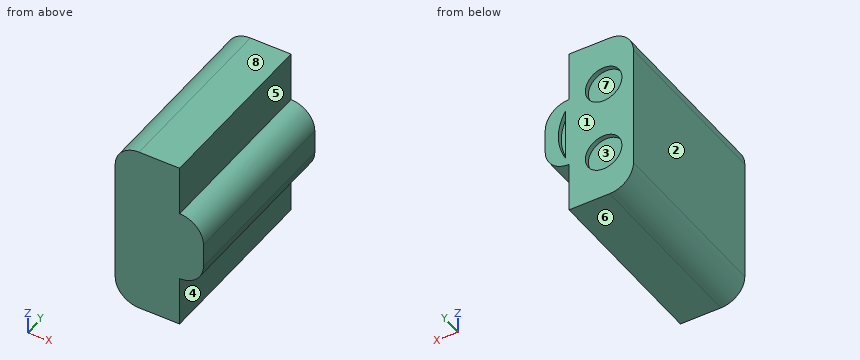
Autodesk Inventor part; units mm, degrees
ref_plane "YZ Plane" through (0, 0, 0) normal (1, 0, 0) x (0, 1, 0)
ref_plane "XZ Plane" through (0, 0, 0) normal (0, 1, 0) x (-1, 0, 0)
ref_plane "XY Plane" through (0, 0, 0) normal (0, 0, 1) x (1, 0, 0)
sketch "Esquisse1" plane through (0, 0, 0) normal (0, 1, 0) x (-1, 0, 0)
  line L0 (0, 0) -> (27, 0)
  line L1 (27, 0) -> (27, -72)
  line L2 (27, -72) -> (0, -72)
  line L3 (0, -72) -> (0, 0)
  line L4 (0, -21) -> (-10, -21)
  line L5 (-10, -21) -> (-10, -51)
  line L6 (-10, -51) -> (0, -51)
  line L7 (0, -51) -> (0, -21)
  point P0 (0, -36)
  dimension "d0" = 27
  dimension "d1" = 72
  dimension "d2" = 30
  dimension "d3" = 10
extrude "Extrusion1" add sketch "Esquisse1" along normal blind 75
sketch "Esquisse2" plane through (0, 75, 0) normal (0, 1, 0) x (1, 0, 0)
  line L0 (0, 21) -> (10, 21) construction
  line L1 (10, 21) -> (10, 51) construction
  line L2 (10, 51) -> (0, 51) construction
  line L3 (0, 51) -> (0, 72) construction
  line L4 (0, 72) -> (-27, 72) construction
  line L5 (-27, 72) -> (-27, 0) construction
  line L6 (-27, 0) -> (0, 0) construction
  line L7 (0, 0) -> (0, 21) construction
  line L8 (-27, 72) -> (-27, 0) construction
  line L9 (-27, 72) -> (-27, 0) construction
  line L10 (-27, 36) -> (10, 36) construction
  circle A0 centre (-14.5005, 20.2664) radius 7.6563
  circle A1 centre (-14.5005, 51.7336) radius 7.6563
  line L11 (1.4504, 25.5678) -> (1.4504, 47.6136)
  line L12 (1.4504, 25.5678) -> (7.5686, 36) construction
  line L13 (7.5686, 36) -> (1.4504, 47.6136) construction
  spline S0 degree 2 poles (1.4504, 25.5678) (7.5686, 36) (1.4504, 47.6136) knots 1 1 1 2 2 2
  dimension "d28" = 15.3126
extrude "Extrusion2" cut sketch "Esquisse2" against normal blind 2
fillet "Congé1" radius 10 2 edges at (-27, 37.5, -72) (-27, 37.5, 0)
fillet "Congé2" radius 10 2 edges at (10, 37.5, -51) (10, 37.5, -21)
ref_plane "Plan de construction1" through (0, 60, 0) normal (0, 1, 0) x (1, 0, 0)
sketch "Esquisse3" plane through (0, 0, -72) normal (0, 0, -1) x (-1, 0, 0)
  point P0 (0, 0)
sketch "Esquisse4" plane through (0, 60, 0) normal (0, 1, 0) x (1, 0, 0)
  arc A0 (0, 21) -> (10, 31) centre (0, 31) ccw
  line L0 (10, 31) -> (10, 41)
  arc A1 (10, 41) -> (0, 51) centre (0, 41) ccw
  line L1 (0, 51) -> (0, 72)
  line L2 (0, 72) -> (-17, 72)
  arc A2 (-17, 72) -> (-27, 62) centre (-17, 62) ccw
  line L3 (-27, 62) -> (-27, 10)
  arc A3 (-27, 10) -> (-17, 0) centre (-17, 10) ccw
  line L4 (-17, 0) -> (0, 0)
  line L5 (0, 0) -> (0, 21)
  circle A4 centre (-14.5005, 20.2664) radius 7.6563
  line L6 (1.4504, 25.5678) -> (1.4504, 47.6136)
  circle A5 centre (-14.5005, 51.7336) radius 7.6563
  line L7 (0, 72) -> (-17, 72)
  line L8 (-14.5005, 72) -> (-37.6894, 78.8251)
  line L9 (-37.6894, 78.8251) -> (-26.0949, 60.5542)
  line L10 (-26.0949, 60.5542) -> (-14.5005, 72)
ref_plane "Plan de construction2" through (0, 0, -36) normal (0, 0, -1) x (-1, 0, 0)
properties part number "head2"
Design review of the part built by this model. Coordinates are the model's own, in mm. Face numbers are marked on the shaded views. A direction names the side the tool comes from. Coordinates: 2 decimals unless noted, no trailing zeros. Write each loop counter-clockwise with the first axis right and the second up, starting at its lowest first coordinate (ties: lowest second). Pieces come first, ordered by that corner, then holes.
1) Machinability: for the marked faces 4, 5, 6, 7 and 8, which of the approach directions +Z, -Z, +X, -X, +Y, -Y give a long, thin tool a straight path to every point of the face, cutting with its end or side? Answer none if there is none.
2) Insertion check: pin 1 (10.5 mm diameter, centred on y = 52.5, z = -63.5, fed in from +X); pin 2 (1.5 mm diameter, centred on x = -15, z = -50, fed in from +Y); pin 3 (1 mm diameter, centred on x = -21, y = 47.5, fed in from +Z). Each pin has a flat end and moves straight along its axis. Give the tip position at first contact, or say it passes through.
3) Mouldability with a two-part tool opening along X and no side actions: class the marked faces 1, 2 and 3 as +X half, -X half, draft (parallel to the pull), parting line (faces both ways), or undercut.
4) To check wall thickness, follow L1, parallel to Y at x = -20, z = -23; L2, parallel to X at y = 67.5, z = -12; L3, parallel to X at y = 33, z = -30.5. State the ranges of each line that lie inside material, in increasing order.
5) Add section B-B (z = -18). Write out the cut boundary in (x, y).
6) Add section C-C (z = -5.5). Write out the cut boundary in (x, y).
Check result:
1. face 4: -Z, +X, +Y, -Y
1. face 5: +Z, +X, +Y, -Y
1. face 6: -Z, +X, -X, +Y, -Y
1. face 7: +Y
1. face 8: +Z, +X, -X, +Y, -Y
2. pin 1: stops at x = 0
2. pin 2: stops at y = 73
2. pin 3: stops at z = -0.63
3. face 1: draft
3. face 2: -X half
3. face 3: undercut
4. L1: y = 0 to 73
4. L2: x = -27 to 0
4. L3: x = -27 to 9.99
5. outline: (-27, 0) - (0, 0) - (0, 75) - (-7.19, 75) - (-7.19, 73) - (-21.81, 73) - (-21.81, 75) - (-27, 75) - close
6. outline: (-25.93, 0) - (0, 0) - (0, 75) - (-25.93, 75) - close
